Read the model definition and answer for the solid it produces. Units are mm, in the model's axes. Face numbers are marked on the shaded views. A direction names the side the tool comes from. Round coordinates to 2 decimals unless told otherwise and drop trailing zeros. Order: outer loops, then holes, each group sorted by start corner. A loop starts at its lowest first (then second) coordinate and runs counter-clockwise, first axis right, second up. Notation, with made-up numbers: M 15,19 L 38,19 A13 ccw 38,25 Z; hole C -34,7.5 d11. An arc over 180 degrees is marked long. Answer as CSV lines item,"result".
```python
from build123d import *

# Parameters (mm, degrees)
F0_W         = 19.05
F0_H         = 4.7625
F0_R         = 12.7
F1_DEPTH     = 6.35
F2_R         = 0.508
F3_T1_DEPTH  = 5.334
F3_T6_ANGLE  = 233.2969892374
F3_T11_ANGLE = 233.2969892374
F3_T16_ANGLE = 233.2969892374
F3_T21_ANGLE = 233.2969892374
F3_T26_ANGLE = 233.2969892374
F3_T31_ANGLE = 233.2969892374
F3_T36_ANGLE = 233.2969892374
F3_T41_ANGLE = 233.2969892374
F3_T46_ANGLE = 233.2969892374
F3_T51_ANGLE = 233.2969892374
F3_T56_ANGLE = 233.2969892374
F3_T61_ANGLE = 233.2969892374
F3_T66_ANGLE = 233.2969892374
F3_T71_ANGLE = 233.2969892374
F3_T76_ANGLE = 233.2969892374
F3_T81_ANGLE = 233.2969892374


# Not quite as in the source:
# - a fillet or chamfer that OpenCascade refuses, or shapes differently, is made with other operations: its cross-section is extruded or revolved along the edge and cut away or added


with BuildPart() as f1:
    # F0 (on Top) → F1 (new body)
    with BuildSketch(Plane.XY):
        with BuildLine():
            Line((17.4625, -42.8625), (17.4625, 0))
            ThreePointArc((17.4625, 0), (0, 17.4625), (-17.4625, 0))
            Line((-17.4625, 0), (-17.4625, -42.8625))
            ThreePointArc((-17.4625, -42.8625), (-15.6026280605, -47.3526280605), (-11.1125, -49.2125))
            Line((-11.1125, -49.2125), (11.1125, -49.2125))
            ThreePointArc((11.1125, -49.2125), (15.6026280605, -47.3526280605), (17.4625, -42.8625))
        make_face()
        with Locations((0, -40.48125)):
            Rectangle(F0_W, F0_H, mode=Mode.SUBTRACT)
        with Locations((0, -21.43125)):
            Rectangle(F0_W, F0_H, mode=Mode.SUBTRACT)
        Circle(F0_R, mode=Mode.SUBTRACT)
    extrude(amount=F1_DEPTH)

    # F2
    f2_edges = [f1.edges().sort_by_distance(p)[0] for p in [
        (0, -23.8125, 6.35),
        (0, -23.8125, 0),
        (0, -19.05, 6.35),
        (0, -38.1, 6.35),
        (0, -42.8625, 6.35),
        (0, -38.1, 0),
        (0, -19.05, 0),
        (0, -42.8625, 0),
    ]]
    fillet(f2_edges, radius=F2_R)

    # F3: fillet of radius 0.508 on 8 edges, made by hand

    # F3_s2 → F3_t1 (join)
    with BuildSketch(Plane.XY.offset(0.508)):
        with BuildLine():
            ThreePointArc((9.525, -42.3545), (9.3762102448, -42.7137102448), (9.017, -42.8625))
            Line((9.017, -42.8625), (9.525, -42.8625))
            Line((9.525, -42.8625), (9.525, -42.3545))
        make_face()
        with BuildLine():
            ThreePointArc((9.525, -23.3045), (9.3762102448, -23.6637102448), (9.017, -23.8125))
            Line((9.017, -23.8125), (9.525, -23.8125))
            Line((9.525, -23.8125), (9.525, -23.3045))
        make_face()
        with BuildLine():
            ThreePointArc((-9.525, -42.3545), (-9.3762102448, -42.7137102448), (-9.017, -42.8625))
            Line((-9.017, -42.8625), (-9.525, -42.8625))
            Line((-9.525, -42.8625), (-9.525, -42.3545))
        make_face()
        with BuildLine():
            ThreePointArc((9.525, -19.558), (9.3762102448, -19.1987897552), (9.017, -19.05))
            Line((9.017, -19.05), (9.525, -19.05))
            Line((9.525, -19.05), (9.525, -19.558))
        make_face()
        with BuildLine():
            ThreePointArc((-9.525, -19.558), (-9.3762102448, -19.1987897552), (-9.017, -19.05))
            Line((-9.017, -19.05), (-9.525, -19.05))
            Line((-9.525, -19.05), (-9.525, -19.558))
        make_face()
        with BuildLine():
            ThreePointArc((-9.525, -23.3045), (-9.3762102448, -23.6637102448), (-9.017, -23.8125))
            Line((-9.017, -23.8125), (-9.525, -23.8125))
            Line((-9.525, -23.8125), (-9.525, -23.3045))
        make_face()
        with BuildLine():
            ThreePointArc((-9.017, -38.1), (-9.3762102448, -38.2487897552), (-9.525, -38.608))
            Line((-9.525, -38.608), (-9.525, -38.1))
            Line((-9.525, -38.1), (-9.017, -38.1))
        make_face()
        with BuildLine():
            ThreePointArc((9.017, -38.1), (9.3762102448, -38.2487897552), (9.525, -38.608))
            Line((9.525, -38.608), (9.525, -38.1))
            Line((9.525, -38.1), (9.017, -38.1))
        make_face()
    extrude(amount=F3_T1_DEPTH)


with BuildPart() as f3_tool4:
    # F3_s5 → F3_t6 (revolve)
    with BuildSketch(Plane.XY.offset(0.508)):
        with BuildLine():
            ThreePointArc((9.017, -38.1), (9.3762102448, -38.2487897552), (9.525, -38.608))
            Line((9.525, -38.608), (9.525, -38.1))
            Line((9.525, -38.1), (9.017, -38.1))
        make_face()
    revolve(axis=Axis((9.525, -37.592, 0.508), (1, 0, 0)), revolution_arc=F3_T6_ANGLE)

    split(bisect_by=Plane.XY, keep=Keep.TOP)


with BuildPart() as f1_1:
    add(f1.part)

    # F3_t3: union F3_tool4
    add(f3_tool4.part)


with BuildPart() as f3_tool9:
    # F3_s10 → F3_t11 (revolve)
    with BuildSketch(Plane.XY.offset(5.842)):
        with BuildLine():
            ThreePointArc((9.017, -38.1), (9.3762102448, -38.2487897552), (9.525, -38.608))
            Line((9.525, -38.608), (9.525, -38.1))
            Line((9.525, -38.1), (9.017, -38.1))
        make_face()
    revolve(axis=Axis((9.525, -37.592, 5.842), (-1, 0, 0)), revolution_arc=F3_T11_ANGLE)

    split(bisect_by=Plane.XY.offset(6.35), keep=Keep.BOTTOM)


with BuildPart() as f1_2:
    add(f1_1.part)

    # F3_t8: union F3_tool9
    add(f3_tool9.part)


with BuildPart() as f3_tool14:
    # F3_s15 → F3_t16 (revolve)
    with BuildSketch(Plane.XY.offset(0.508)):
        with BuildLine():
            ThreePointArc((-9.525, -38.608), (-9.3762102448, -38.2487897552), (-9.017, -38.1))
            Line((-9.017, -38.1), (-9.525, -38.1))
            Line((-9.525, -38.1), (-9.525, -38.608))
        make_face()
    revolve(axis=Axis((-9.525, -37.592, 0.508), (1, 0, 0)), revolution_arc=F3_T16_ANGLE)

    split(bisect_by=Plane.XY, keep=Keep.TOP)


with BuildPart() as f1_3:
    add(f1_2.part)

    # F3_t13: union F3_tool14
    add(f3_tool14.part)


with BuildPart() as f3_tool19:
    # F3_s20 → F3_t21 (revolve)
    with BuildSketch(Plane.XY.offset(5.842)):
        with BuildLine():
            ThreePointArc((-9.525, -38.608), (-9.3762102448, -38.2487897552), (-9.017, -38.1))
            Line((-9.017, -38.1), (-9.525, -38.1))
            Line((-9.525, -38.1), (-9.525, -38.608))
        make_face()
    revolve(axis=Axis((-9.525, -37.592, 5.842), (-1, 0, 0)), revolution_arc=F3_T21_ANGLE)

    split(bisect_by=Plane.XY.offset(6.35), keep=Keep.BOTTOM)


with BuildPart() as f1_4:
    add(f1_3.part)

    # F3_t18: union F3_tool19
    add(f3_tool19.part)


with BuildPart() as f3_tool24:
    # F3_s25 → F3_t26 (revolve)
    with BuildSketch(Plane.XY.offset(0.508)):
        with BuildLine():
            ThreePointArc((-9.017, -23.8125), (-9.3762102448, -23.6637102448), (-9.525, -23.3045))
            Line((-9.525, -23.3045), (-9.525, -23.8125))
            Line((-9.525, -23.8125), (-9.017, -23.8125))
        make_face()
    revolve(axis=Axis((-9.525, -24.3205, 0.508), (-1, 0, 0)), revolution_arc=F3_T26_ANGLE)

    split(bisect_by=Plane.XY, keep=Keep.TOP)


with BuildPart() as f1_5:
    add(f1_4.part)

    # F3_t23: union F3_tool24
    add(f3_tool24.part)


with BuildPart() as f3_tool29:
    # F3_s30 → F3_t31 (revolve)
    with BuildSketch(Plane.XY.offset(5.842)):
        with BuildLine():
            ThreePointArc((-9.525, -23.3045), (-9.3762102448, -23.6637102448), (-9.017, -23.8125))
            Line((-9.017, -23.8125), (-9.525, -23.8125))
            Line((-9.525, -23.8125), (-9.525, -23.3045))
        make_face()
    revolve(axis=Axis((-9.525, -24.3205, 5.842), (1, 0, 0)), revolution_arc=F3_T31_ANGLE)

    split(bisect_by=Plane.XY.offset(6.35), keep=Keep.BOTTOM)


with BuildPart() as f1_6:
    add(f1_5.part)

    # F3_t28: union F3_tool29
    add(f3_tool29.part)


with BuildPart() as f3_tool34:
    # F3_s35 → F3_t36 (revolve)
    with BuildSketch(Plane.XY.offset(0.508)):
        with BuildLine():
            ThreePointArc((-9.525, -19.558), (-9.3762102448, -19.1987897552), (-9.017, -19.05))
            Line((-9.017, -19.05), (-9.525, -19.05))
            Line((-9.525, -19.05), (-9.525, -19.558))
        make_face()
    revolve(axis=Axis((-9.525, -18.542, 0.508), (1, 0, 0)), revolution_arc=F3_T36_ANGLE)

    split(bisect_by=Plane.XY, keep=Keep.TOP)


with BuildPart() as f1_7:
    add(f1_6.part)

    # F3_t33: union F3_tool34
    add(f3_tool34.part)


with BuildPart() as f3_tool39:
    # F3_s40 → F3_t41 (revolve)
    with BuildSketch(Plane.XY.offset(5.842)):
        with BuildLine():
            ThreePointArc((-9.525, -19.558), (-9.3762102448, -19.1987897552), (-9.017, -19.05))
            Line((-9.017, -19.05), (-9.525, -19.05))
            Line((-9.525, -19.05), (-9.525, -19.558))
        make_face()
    revolve(axis=Axis((-9.525, -18.542, 5.842), (-1, 0, 0)), revolution_arc=F3_T41_ANGLE)

    split(bisect_by=Plane.XY.offset(6.35), keep=Keep.BOTTOM)


with BuildPart() as f1_8:
    add(f1_7.part)

    # F3_t38: union F3_tool39
    add(f3_tool39.part)


with BuildPart() as f3_tool44:
    # F3_s45 → F3_t46 (revolve)
    with BuildSketch(Plane.XY.offset(0.508)):
        with BuildLine():
            ThreePointArc((9.525, -19.558), (9.3762102448, -19.1987897552), (9.017, -19.05))
            Line((9.017, -19.05), (9.525, -19.05))
            Line((9.525, -19.05), (9.525, -19.558))
        make_face()
    revolve(axis=Axis((9.525, -18.542, 0.508), (1, 0, 0)), revolution_arc=F3_T46_ANGLE)

    split(bisect_by=Plane.XY, keep=Keep.TOP)


with BuildPart() as f1_9:
    add(f1_8.part)

    # F3_t43: union F3_tool44
    add(f3_tool44.part)


with BuildPart() as f3_tool49:
    # F3_s50 → F3_t51 (revolve)
    with BuildSketch(Plane.XY.offset(5.842)):
        with BuildLine():
            ThreePointArc((9.525, -19.558), (9.3762102448, -19.1987897552), (9.017, -19.05))
            Line((9.017, -19.05), (9.525, -19.05))
            Line((9.525, -19.05), (9.525, -19.558))
        make_face()
    revolve(axis=Axis((9.525, -18.542, 5.842), (-1, 0, 0)), revolution_arc=F3_T51_ANGLE)

    split(bisect_by=Plane.XY.offset(6.35), keep=Keep.BOTTOM)


with BuildPart() as f1_10:
    add(f1_9.part)

    # F3_t48: union F3_tool49
    add(f3_tool49.part)


with BuildPart() as f3_tool54:
    # F3_s55 → F3_t56 (revolve)
    with BuildSketch(Plane.XY.offset(0.508)):
        with BuildLine():
            ThreePointArc((-9.525, -42.3545), (-9.3762102448, -42.7137102448), (-9.017, -42.8625))
            Line((-9.017, -42.8625), (-9.525, -42.8625))
            Line((-9.525, -42.8625), (-9.525, -42.3545))
        make_face()
    revolve(axis=Axis((-9.525, -43.3705, 0.508), (-1, 0, 0)), revolution_arc=F3_T56_ANGLE)

    split(bisect_by=Plane.XY, keep=Keep.TOP)


with BuildPart() as f1_11:
    add(f1_10.part)

    # F3_t53: union F3_tool54
    add(f3_tool54.part)


with BuildPart() as f3_tool59:
    # F3_s60 → F3_t61 (revolve)
    with BuildSketch(Plane.XY.offset(5.842)):
        with BuildLine():
            ThreePointArc((-9.525, -42.3545), (-9.3762102448, -42.7137102448), (-9.017, -42.8625))
            Line((-9.017, -42.8625), (-9.525, -42.8625))
            Line((-9.525, -42.8625), (-9.525, -42.3545))
        make_face()
    revolve(axis=Axis((-9.525, -43.3705, 5.842), (1, 0, 0)), revolution_arc=F3_T61_ANGLE)

    split(bisect_by=Plane.XY.offset(6.35), keep=Keep.BOTTOM)


with BuildPart() as f1_12:
    add(f1_11.part)

    # F3_t58: union F3_tool59
    add(f3_tool59.part)


with BuildPart() as f3_tool64:
    # F3_s65 → F3_t66 (revolve)
    with BuildSketch(Plane.XY.offset(0.508)):
        with BuildLine():
            ThreePointArc((9.525, -23.3045), (9.3762102448, -23.6637102448), (9.017, -23.8125))
            Line((9.017, -23.8125), (9.525, -23.8125))
            Line((9.525, -23.8125), (9.525, -23.3045))
        make_face()
    revolve(axis=Axis((9.525, -24.3205, 0.508), (-1, 0, 0)), revolution_arc=F3_T66_ANGLE)

    split(bisect_by=Plane.XY, keep=Keep.TOP)


with BuildPart() as f1_13:
    add(f1_12.part)

    # F3_t63: union F3_tool64
    add(f3_tool64.part)


with BuildPart() as f3_tool69:
    # F3_s70 → F3_t71 (revolve)
    with BuildSketch(Plane.XY.offset(5.842)):
        with BuildLine():
            ThreePointArc((9.525, -23.3045), (9.3762102448, -23.6637102448), (9.017, -23.8125))
            Line((9.017, -23.8125), (9.525, -23.8125))
            Line((9.525, -23.8125), (9.525, -23.3045))
        make_face()
    revolve(axis=Axis((9.525, -24.3205, 5.842), (1, 0, 0)), revolution_arc=F3_T71_ANGLE)

    split(bisect_by=Plane.XY.offset(6.35), keep=Keep.BOTTOM)


with BuildPart() as f1_14:
    add(f1_13.part)

    # F3_t68: union F3_tool69
    add(f3_tool69.part)


with BuildPart() as f3_tool74:
    # F3_s75 → F3_t76 (revolve)
    with BuildSketch(Plane.XY.offset(0.508)):
        with BuildLine():
            ThreePointArc((9.525, -42.3545), (9.3762102448, -42.7137102448), (9.017, -42.8625))
            Line((9.017, -42.8625), (9.525, -42.8625))
            Line((9.525, -42.8625), (9.525, -42.3545))
        make_face()
    revolve(axis=Axis((9.525, -43.3705, 0.508), (-1, 0, 0)), revolution_arc=F3_T76_ANGLE)

    split(bisect_by=Plane.XY, keep=Keep.TOP)


with BuildPart() as f1_15:
    add(f1_14.part)

    # F3_t73: union F3_tool74
    add(f3_tool74.part)


with BuildPart() as f3_tool79:
    # F3_s80 → F3_t81 (revolve)
    with BuildSketch(Plane.XY.offset(5.842)):
        with BuildLine():
            ThreePointArc((9.525, -42.3545), (9.3762102448, -42.7137102448), (9.017, -42.8625))
            Line((9.017, -42.8625), (9.525, -42.8625))
            Line((9.525, -42.8625), (9.525, -42.3545))
        make_face()
    revolve(axis=Axis((9.525, -43.3705, 5.842), (1, 0, 0)), revolution_arc=F3_T81_ANGLE)

    split(bisect_by=Plane.XY.offset(6.35), keep=Keep.BOTTOM)


with BuildPart() as f1_16:
    add(f1_15.part)

    # F3_t78: union F3_tool79
    add(f3_tool79.part)


solid = f1_16.part
```
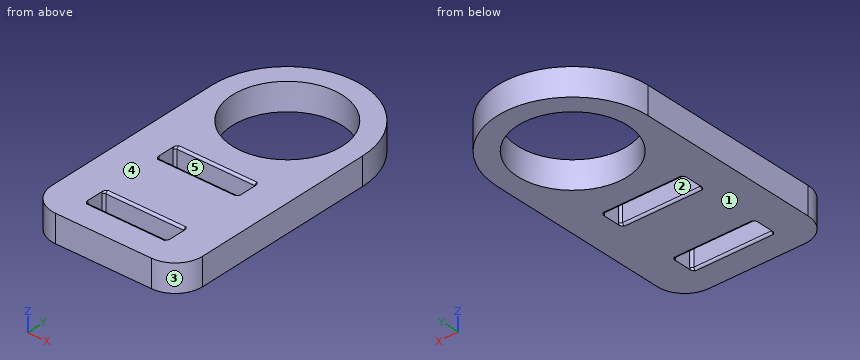
Item 1: A cutting plane is placed at B-B, the plane z = 3. Give the number of separate pieces and of enclosed holes in the cut face, and give its area (3 significant figures).
Ans:
separate pieces,"1"
enclosed holes,"3"
area,"1,490 mm2"
Item 2: Find the intervals of material crossed by probe 1 along Y at (x, z) = (0, 4.75); probe 2 along X at (y, z) = (-39.5, 5.5) (1 decimal); probe 3 along Y at (x, z) = (2.5, 6), in increasing order. Write a range as [from, to].
Ans:
probe 1,"[-49.21, -42.86], [-38.1, -23.81], [-19.05, -12.7], [12.7, 17.46]"
probe 2,"[-17.5, -9.5], [9.5, 17.5]"
probe 3,"[-49.21, -42.89], [-38.07, -23.84], [-19.02, -12.45], [12.45, 17.28]"
Item 3: A flat-ended cylindrical pin translates along its axis: pin 1 (1 mm diameter, centred on x = -12.5, z = 3, fed in from +Y). Find the tip coordinate at first contact, or state that the pin passes through.
Ans:
pin 1,"y = 12.69"
Item 4: A cutting plane is placed at C-C, the plane y = 12. Determine the outline of the cut face in (x, z).
Ans:
outline,"M -12.69,0 L -4.16,0 L -4.16,6.35 L -12.69,6.35 Z; M 4.16,0 L 12.69,0 L 12.69,6.35 L 4.16,6.35 Z"
Item 5: A tool of negligible diameter and unlimited length cuts with its end or side. For the marked faces 4 and 5, from which of +Z, -Z, +X, -X, +Y, -Y can it reach the whole face along a straight path? Write none if from no direction.
Ans:
face 4,"+Z, +X, -X, +Y, -Y"
face 5,"+Z, -Z"
Item 6: A cutting plane is placed at A-A, the plane x = 0. Determine the outline of the cut face in (y, z).
Ans:
outline,"M -49.21,0 L -43.37,0 A0.51 ccw -42.86,0.51 L -42.86,5.84 A0.51 ccw -43.37,6.35 L -49.21,6.35 Z; M -38.1,0.51 A0.51 ccw -37.59,0 L -24.32,0 A0.51 ccw -23.81,0.51 L -23.81,5.84 A0.51 ccw -24.32,6.35 L -37.59,6.35 A0.51 ccw -38.1,5.84 Z; M -19.05,0.51 A0.51 ccw -18.54,0 L -12.7,0 L -12.7,6.35 L -18.54,6.35 A0.51 ccw -19.05,5.84 Z; M 12.7,0 L 17.46,0 L 17.46,6.35 L 12.7,6.35 Z"
Item 7: A cutting plane is placed at D-D, the plane x = -6. Determine the outline of the cut face in (y, z), and give its area (3 significant figures).
Ans:
outline,"M -49.21,0 L -43.37,0 A0.51 ccw -42.86,0.51 L -42.86,5.84 A0.51 ccw -43.37,6.35 L -49.21,6.35 Z; M -38.1,0.51 A0.51 ccw -37.59,0 L -24.32,0 A0.51 ccw -23.81,0.51 L -23.81,5.84 A0.51 ccw -24.32,6.35 L -37.59,6.35 A0.51 ccw -38.1,5.84 Z; M -19.05,0.51 A0.51 ccw -18.54,0 L -11.19,0 L -11.19,6.35 L -18.54,6.35 A0.51 ccw -19.05,5.84 Z; M 11.19,0 L 16.4,0 L 16.4,6.35 L 11.19,6.35 Z"
area,"214 mm2"
Item 8: Determine the mould class of the marked faces 1, 2 and 3 for opening direction Y: +Y half, -Y half, draft (parallel to the pull), parting line (faces both ways), or undercut.
Ans:
face 1,"draft"
face 2,"undercut"
face 3,"-Y half"
